Could you check a few things on this drawing? It's one solid part, dimensions in mm from its lowest x, y, z. A direction names the side the tool comes from. Give positions to 0.01 mm unless a question says otherwise; leave off trailing zeros. Loops run counter-clockwise (first coordinate to the right, second up) from the corner with the lowest first, then second, coordinate; pieces in that order, holes last. Notation, with made-up numbers: M 71.25,68.25 L 95.25,68.25 A19 ccw 95.25,75.25 Z; hole C -10.5,-9.5 d2. An arc over 180 degrees is marked long. One line per item, written item: value. Start each with the question number.
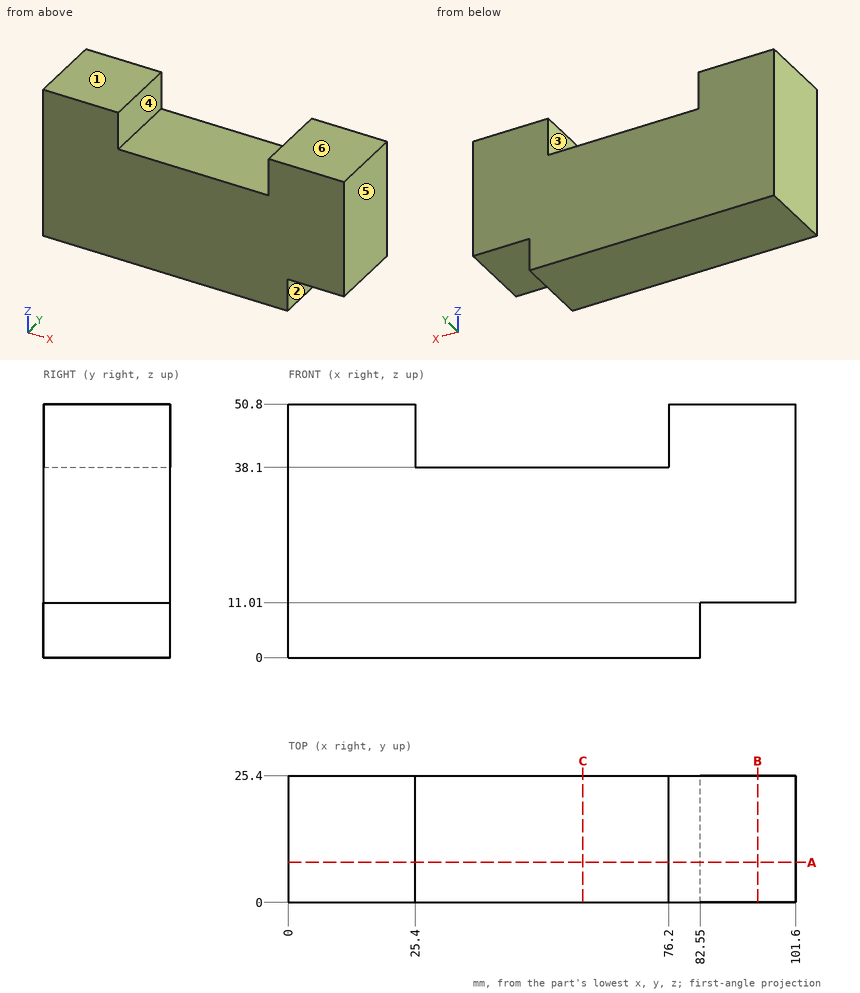
Q1. If we section it at B-B, the plane x = 94: Write out the boundary of the cut face in (y, z).
Q2. If we mould it in two halves opening along X, with no side actions, what happens to the marked faces 4, 5 and 6? For each: released by +X, released by -X, zero draft, split by the parting line, or undercut.
Q3. If we section it at C-C, the plane x = 59: Write out the boundary of the cut face in (y, z).
Q4. If we section it at A-A, the plane y = 8: Write out the boundary of the cut face in (x, z), plus the area to 3 significant figures.
Q5. Which directions (+Z, -Z, +X, -X, +Y, -Y) give clear straight access to the entire face, cutting with the end or side of a thin tool? Please do the marked faces 1, 2 and 3.
Q6. For P1, Ø14, axis at y = 8.5, z = 47.5, coming from the -X side; P2, Ø1.5, axis at x = 42.5, y = 18, coming from the +Z side; P3, Ø5.5, axis at y = 8, z = 4.5, coming from the +X side; P4, Ø5.5, axis at x = 92, y = 14, coming from the -Z side, each with a flat end and sliding along its axis, tell me the tip position at first contact or that it passes through.
Q7. I need wall thicknesses on line 1 along X through (y, z) = (23.5, 42.5); line 2 along Z through (x, y) = (29, 4); line 3 along Z through (x, y) = (83, 10.5). Which ranges of each line are inside material? Lowest first, please.
Response:
1. outline: M 0,11.01 L 25.4,11.01 L 25.4,50.8 L 0,50.8 Z
2. face 4: undercut
2. face 5: released by +X
2. face 6: zero draft
3. outline: M 0,0 L 25.4,0 L 25.4,38.1 L 0,38.1 Z
4. outline: M 0,0 L 82.55,0 L 82.55,11.01 L 101.6,11.01 L 101.6,50.8 L 76.2,50.8 L 76.2,38.1 L 25.4,38.1 L 25.4,50.8 L 0,50.8 Z
4. area: 4,310 mm^2
5. face 1: +Z, +X, -X, +Y, -Y
5. face 2: -Z, +X, +Y, -Y
5. face 3: +Z, +Y, -Y
6. P1: x = 0
6. P2: z = 38.1
6. P3: x = 82.55
6. P4: z = 11.01
7. line 1: 0 to 25.4, 76.2 to 101.6
7. line 2: 0 to 38.1
7. line 3: 11.01 to 50.8
